from build123d import *

# Parameters (mm, degrees)
F1_DEPTH = 40
F2_R     = 10
F3_R     = 1.5
F4_DEPTH = 6
F5_W     = 11
F5_H     = 7.0209084079
F6_DEPTH = 5
F7_W     = 3.1
F7_H     = 9
F8_DEPTH = 25


with BuildPart() as f1:
    # F0 (on Front) → F1 (new body)
    with BuildSketch(Plane.XZ):
        Polygon((-5, 15), (-5, 0), (-35, 0), (-35, -2), (-5, -2), (0, -2), (0, 0), (0, 15), align=None)
    extrude(amount=F1_DEPTH)

    # F2
    f2_edges = [f1.edges().sort_by_distance(p)[0] for p in [
        (-5, -20, 0),
    ]]
    fillet(f2_edges, radius=F2_R)

    # F3 (on face) → F4 (cut)
    with BuildSketch(Plane.XY):
        with Locations((-30, -9.5)):
            Circle(F3_R)
        with Locations((-30, -29.4)):
            Circle(F3_R)
    extrude(amount=-F4_DEPTH, mode=Mode.SUBTRACT)

    # F5 (on face) → F6 (join)
    with BuildSketch(Plane.YZ):
        with Locations((-20, 9.9406884983)):
            Rectangle(F5_W, F5_H)
    extrude(amount=F6_DEPTH)

    # F7 (on face) → F8 (cut)
    with BuildSketch(Plane.XY.offset(13.4511427023)):
        with Locations((2.5, -20)):
            Rectangle(F7_W, F7_H)
    extrude(amount=-F8_DEPTH, mode=Mode.SUBTRACT)


solid = f1.part
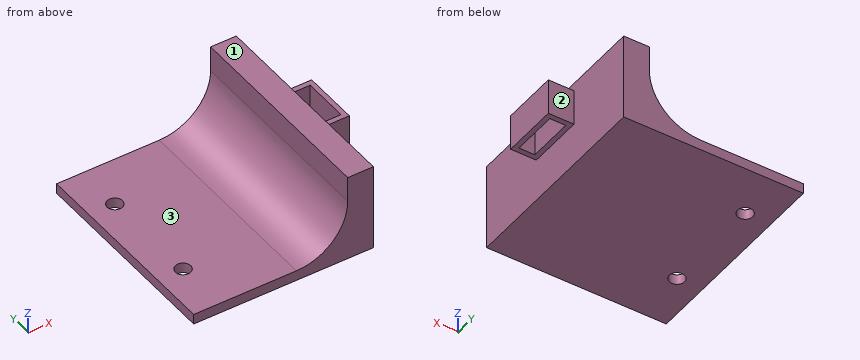
Geometry check sheet. Reference: the model listing, model coordinates, mm. Face numbers are marked on the shaded views. A direction names the side the tool comes from. Round coordinates to 2 decimals unless told otherwise and drop trailing zeros. Write each loop counter-clockwise with the first axis right and the second up, starting at its lowest first coordinate (ties: lowest second). Pieces come first, ordered by that corner, then holes.
Item 1: Section check D-D (y = -32). Record the boundary of the cut face in (x, z), plus the area to 3 significant figures.
Determined:
outline: (-35, -2) - (0, -2) - (0, 15) - (-5, 15) - (-5, 10) arc R10 cw to (-15, 0) - (-35, 0) - close
area: 166 mm2
Item 2: Material ranges on line 1 along Y through (x, z) = (-30, -1.25); line 2 along Z through (x, y) = (-20.5, -19.5); line 3 along X through (y, z) = (-27, 13), recorded low to high.
Determined:
line 1: y = -40 to -30.9, -27.9 to -11, -8 to 0
line 2: z = -2 to 0
line 3: x = -5 to 0
Item 3: Go/stop test with flat-tipped pins: pin 1 Ø2.5 at (x, y) = (2.5, -22.5) entering from -Z; pin 2 Ø3.5 at (x, y) = (-30, -29.4) entering from +Z; pin 3 Ø3.5 at (x, z) = (2, 9.5) entering from +Y; pin 4 Ø2 at (y, z) = (-18, 11.5) entering from -X. Record where each tip stops, or that it passes through.
Determined:
pin 1: passes through
pin 2: stops at z = 0
pin 3: stops at y = -14.5
pin 4: stops at x = -5
Item 4: Section check A-A (x = -30). Record the boundary of the cut face in (y, z).
Determined:
outline: (-40, -2) - (-30.9, -2) - (-30.9, 0) - (-40, 0) - close; (-27.9, -2) - (-11, -2) - (-11, 0) - (-27.9, 0) - close; (-8, -2) - (0, -2) - (0, 0) - (-8, 0) - close
Item 5: Section check C-C (z = 11.75). Record the boundary of the cut face in (x, y), plus the area to 3 significant figures.
Determined:
outline: (-5, -40) - (0, -40) - (0, -25.5) - (5, -25.5) - (5, -14.5) - (0, -14.5) - (0, 0) - (-5, 0) - close; hole (0.95, -24.5) - (4.05, -24.5) - (4.05, -15.5) - (0.95, -15.5) - close
area: 227 mm2
Item 6: Section check B-B (y = -9.5). Record the boundary of the cut face in (x, z).
Determined:
outline: (-35, -2) - (-31.5, -2) - (-31.5, 0) - (-35, 0) - close; (-28.5, -2) - (0, -2) - (0, 15) - (-5, 15) - (-5, 10) arc R10 cw to (-15, 0) - (-28.5, 0) - close
Item 7: Access from +Z, -Z, +X, -X, +Y, -Y to the whole of each face (thin tool, end or side, straight path). Record for the marked faces 1, 2 and 3.
Determined:
face 1: +Z, +X, -X, +Y, -Y
face 2: +Z, -Z, +X, +Y
face 3: +Z, -X, +Y, -Y
